Autodesk Inventor part; units mm, degrees
ref_plane "YZ Plane" through (0, 0, 0) normal (1, 0, 0) x (0, 1, 0)
ref_plane "XZ Plane" through (0, 0, 0) normal (0, 1, 0) x (-1, 0, 0)
ref_plane "XY Plane" through (0, 0, 0) normal (0, 0, 1) x (1, 0, 0)
sketch "草圖1" plane through (0, 0, 0) normal (0, 0, 1) x (1, 0, 0)
  line L0 (0, 0) -> (0, 13)
  line L1 (0, 13) -> (14.8465, 17.3666)
  line L2 (17, 20.2447) -> (17, 37.5)
  line L3 (14, 40.5) -> (2, 40.5)
  line L4 (2, 44.5) -> (49, 44.5)
  line L5 (49, 40.5) -> (37, 40.5)
  line L6 (34, 37.5) -> (34, 20.2447)
  line L7 (36.1535, 17.3666) -> (51, 13)
  line L8 (51, 13) -> (51, 0)
  line L9 (51, 0) -> (0, 0)
  line L10 (2, 40.5) -> (2, 44.5)
  line L11 (49, 40.5) -> (49, 44.5)
  line L12 (25.5, 0) -> (25.5, 70.2145)
  arc A0 (14.8465, 17.3666) -> (17, 20.2447) centre (14, 20.2447) ccw
  arc A1 (34, 20.2447) -> (36.1535, 17.3666) centre (37, 20.2447) ccw
  arc A2 (17, 37.5) -> (14, 40.5) centre (14, 37.5) ccw
  arc A3 (37, 40.5) -> (34, 37.5) centre (37, 37.5) ccw
  point P0 (17, 18)
  point P1 (17, 40.5)
  point P2 (34, 40.5)
  point P3 (34, 18)
  dimension "d0" = 51
  dimension "d1" = 47
  dimension "d2" = 17
  dimension "d3" = 18
  dimension "d4" = 4
  dimension "d5" = 40.5
  dimension "d6" = 15
  dimension "d7" = 18
  dimension "d8" = 13
  dimension "d9" = 13
  dimension "d10" = 3
revolve "迴轉1" add sketch "草圖1" angle 180 about axis through (51, 0, 0) along (-1, 0, 0)
sketch "草圖2" plane through (51, 0, 0) normal (1, 0, 0) x (0, 0, -1)
  circle A0 centre (0, 0) radius 6.5
  dimension "d13" = 13
extrude "擠出1" cut sketch "草圖2" against normal up to next
fillet "圓角1" radius 3 2 edges at (51, 0, -13) (0, 0, -13)
properties part number "練習二"
Verification items for the finished model (mm, model axes). A direction names the side the tool comes from. Coordinates: 2 decimals unless noted, no trailing zeros. Order: outer loops, then holes, each group sorted by start corner. A loop starts at its lowest first (then second) coordinate and runs counter-clockwise, first axis right, second up. Notation, with made-up numbers: M 72.5,31 L 84.5,31 A23 cw 84.5,42 Z; hole C 24.25,57 d1. An arc over 180 degrees is marked long. Return JSON: item names as keys, results as strings.
1) Cross-section at B-B, the plane y = 0. Record the boundary of the cut face in (x, z), and give its area (3 significant figures).
Answer list:
{"outline": "M 0,-10.76 A3 ccw 2.15,-13.63 L 14.85,-17.37 A3 cw 17,-20.24 L 17,-37.5 A3 cw 14,-40.5 L 2,-40.5 L 2,-44.5 L 49,-44.5 L 49,-40.5 L 37,-40.5 A3 cw 34,-37.5 L 34,-20.24 A3 cw 36.15,-17.37 L 48.85,-13.63 A3 ccw 51,-10.76 L 51,-6.5 L 0,-6.5 Z", "area": "1,080 mm2"}
2) Access from +Z, -Z, +X, -X, +Y, -Y to the whole of each face (thin tool, end or side, straight path). Record for faces 4 (the conical face through (7.18, -0.33, -15.11)), 5 (the flat face through (51, 0, -7)), 6 (the cylindrical face through (42.92, 0.89, -40.49)).
Answer list:
{"face 4": "-X", "face 5": "+Z, -Z, +X, +Y, -Y", "face 6": "+X"}
3) Thickness scan on L1, parallel to Y at x = 16.5, z = -11.5; L2, parallel to Y at x = 43.5, z = -10; L3, parallel to X at y = 23, z = -15. Record the ranges inside material, lowest first. Write a range as [from, to].
Answer list:
{"L1": "[-42.99, -37.43], [-14.6, 14.6], [37.43, 42.99]", "L2": "[-43.36, -39.25], [-11.46, 11.46], [39.25, 43.36]", "L3": "[17, 34]"}
4) Release check for a two-part mould opening along Y. For faces 1 (the cylindrical face through (25.9, -0.1, -6.5)), 2 (the flat face through (25, -25, 0)), 3 (the cylindrical face through (25.83, -0.98, -44.49)) record: +Y half, -Y half, draft (parallel to the pull), parting line (faces both ways), or undercut.
Answer list:
{"face 1": "undercut", "face 2": "draft", "face 3": "parting line"}
5) Cross-section at D-D, the plane x = 23. Record the boundary of the cut face in (y, z).
Answer list:
{"outline": "M -44.5,0 A44.5 ccw 44.5,0 L 6.5,0 A6.5 cw -6.5,0 Z"}
6) Cross-section at C-C, the plane x = 45.5. Record the boundary of the cut face in (y, z), and give its area (3 significant figures).
Answer list:
{"outline": "M -44.5,0 A44.5 ccw 44.5,0 L 40.5,0 A40.5 cw -40.5,0 Z; M -14.62,0 A14.62 ccw 14.62,0 L 6.5,0 A6.5 cw -6.5,0 Z", "area": "803 mm2"}
7) Cross-section at A-A, the plane x = 8. Record the boundary of the cut face in (y, z).
Answer list:
{"outline": "M -44.5,0 A44.5 ccw 44.5,0 L 40.5,0 A40.5 cw -40.5,0 Z; M -15.35,0 A15.35 ccw 15.35,0 L 6.5,0 A6.5 cw -6.5,0 Z"}
8) Gauge pin test, flat ends, axial feed: pin 1 (22 mm diameter, centred on y = -18.5, z = -14, fed in from +X); pin 2 (10 mm diameter, centred on x = 8, y = 0.5, fed in from +Z); pin 3 (8 mm diameter, centred on x = 39, z = -24.5, fed in from +Y). Record the tip position at first contact, or that the pin passes through.
Answer list:
{"pin 1": "x = 50.63", "pin 2": "z = -3.46", "pin 3": "y = 39.5"}
